Can you work these out from the drawing? Everything is in mm from the part's minimum corner. A direction names the side the tool comes from. Give positions to 0.01 mm unless a question says otherwise; leave off trailing zeros. Order: outer loops, then holes, each group sorted by start corner. A loop starts at its lowest first (then second) coordinate and runs counter-clockwise, first axis right, second up. Notation, with made-up numbers: (72, 80) - (82, 80) arc R21 cw to (82, 91) - close; hole circle Ø11 at (-10.75, -35). An arc over 180 degrees is marked (long way). One line per question, with ' | ' between items.
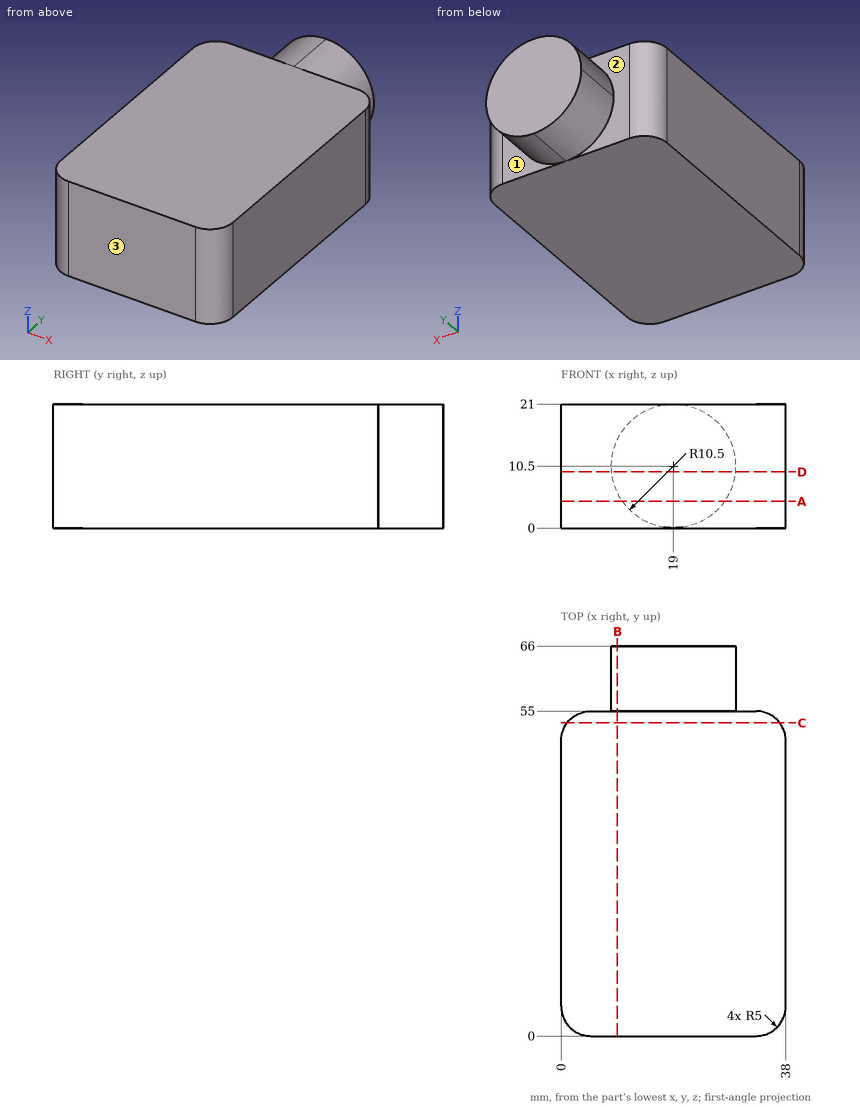
(1) If I drill on line 1 (Y direction, x = 32.5, z = 3); line 2 (Y direction, x = 3, z = 18.5); line 3 (X direction, y = 53.5, z = 7.5), over which ranges is the centre line in solid material (lowest first)?
Answer below:
line 1: 0 to 55 | line 2: 0.42 to 54.58 | line 3: 1.43 to 36.57
(2) Imagine slicing it at B-B (x = 9.5). List the corners of the cut face in (y, z) for me.
Answer below:
outline: (0, 0) - (55, 0) - (55, 6.03) - (66, 6.03) - (66, 14.97) - (55, 14.97) - (55, 21) - (0, 21) - close
(3) Will this pin go through, and if not, where does the flat tip stop? pin 1 (1.5 mm diameter, centred on y = 25.5, z = 9.5, fed in from -X).
Answer below:
pin 1: x = 0
(4) Imagine slicing it at A-A (z = 4.5). List the corners of the cut face in (x, y) for me, and give its area (3 significant figures).
Answer below:
outline: (0, 5) arc R5 ccw to (5, 0) - (33, 0) arc R5 ccw to (38, 5) - (38, 50) arc R5 ccw to (33, 55) - (27.62, 55) - (27.62, 66) - (10.38, 66) - (10.38, 55) - (5, 55) arc R5 ccw to (0, 50) - close | area: 2,260 mm^2
(5) Imagine slicing it at D-D (z = 9.5). List the corners of the cut face in (x, y) for me, and give its area (3 significant figures).
Answer below:
outline: (0, 5) arc R5 ccw to (5, 0) - (33, 0) arc R5 ccw to (38, 5) - (38, 50) arc R5 ccw to (33, 55) - (29.45, 55) - (29.45, 66) - (8.55, 66) - (8.55, 55) - (5, 55) arc R5 ccw to (0, 50) - close | area: 2,300 mm^2
(6) On a 3-axis mill with a long thin cutter (end or side, diameter ignored), from which of +Z, -Z, +X, -X, +Y, -Y can I reach the whole of each face in a straight line? I mean the marked faces 1, 2 and 3. Say none if no direction works.
Answer below:
face 1: +X, +Y | face 2: -X, +Y | face 3: +Z, -Z, +X, -X, -Y
(7) Imagine slicing it at C-C (y = 53). List the corners of the cut face in (x, z) for me.
Answer below:
outline: (1, 0) - (37, 0) - (37, 21) - (1, 21) - close
